Model file for the job. Use its own axes, mm. A direction names the side the tool comes from. Round coordinates to 2 decimals unless told otherwise and drop trailing zeros. Loops run counter-clockwise (first coordinate to the right, second up) from the corner with the lowest first, then second, coordinate; pieces in that order, holes last. Notation, with made-up numbers: M 86.5,-15.5 L 106.5,-15.5 A10 cw 106.5,-8.5 Z; hole C 21,70 d3. An arc over 180 degrees is marked long. Use a Markdown table: item, result. Add a question column.
Q1. Pin check, flat tips, straight feed: pin 1 (2 mm diameter, centred on x = 50, z = 8.5, fed in from -Y); pin 2 (1.4 mm diameter, centred on x = 2, y = 6.5, fed in from +Z); pin 3 (1.6 mm diameter, centred on x = 0.5, z = 12.5, fed in from -Y). Stop position of each tip, or through.
Q2. Cut at A-A (y = 5). Give the cut face in (x, z) (1 decimal).
Q3. Cut at B-B (x = 18). Give the cut face in (y, z), plus the area to 3 significant figures.
Q4. Probe line 1 (X direction, y = 1, z = -0.75); line 2 (Y direction, x = 54, z = -8); line 3 (Y direction, x = 9.5, z = -11). List the from-to ranges inside material, lowest first. Write a range as from..to.
Q5. Tool access for faces 1 (the face through (2, 8, 12)), 2 (the face through (1, 7.3, -12)), 3 (the face through (1, 7.3, 12)): list every direction of +Z, -Z, +X, -X, +Y, -Y with a clear straight run to the whole face (end or side of a thin tool).
Q6. Mould opens along X. For faces 4 (the face through (46.633, 8.243, -0.182)), 5 (the face through (17.99, 12.75, 0.18)), 6 (the face through (60.87, 5.61, 5.48)) say: +X half, -X half, draft (parallel to the pull), parting line (faces both ways), or undercut.
Autodesk Inventor part; units mm, degrees
ref_plane "AK_XY" through (0, -0.05, 0) normal (-1, 0, 0) x (0, 0, -1)
ref_plane "AK_YZ" through (0, -0.05, 0) normal (0, 0, -1) x (0, -1, 0)
ref_plane "AK_ZX" through (0, -0.05, 0) normal (0, -1, 0) x (-1, 0, 0)
sketch "Sketch_26" plane through (0, 0, 0) normal (0, 0, 1) x (1, 0, 0)
  line L0 (0, 15) -> (0, 0)
  line L1 (0, 0) -> (62.6, 0)
  line L2 (62.6, 0) -> (62.6, 15)
  line L3 (62.6, 15) -> (0, 15)
extrude "Extrusion1" add sketch "Sketch_26" along normal mid plane 26
sketch "Sketch_1" plane through (0, 0, 0) normal (1, 0, 0) x (0, 0, -1)
  arc A0 (13, 11.25) -> (-13, 11.25) centre (0, -44.3333) ccw
  line L0 (13, 11.25) -> (13, 20.75)
  line L1 (13, 20.75) -> (-13, 20.75)
  line L2 (-13, 20.75) -> (-13, 11.25)
extrude "Extrusion2" cut sketch "Sketch_1" along normal blind 36.5
sketch "Sketch_12" plane through (0, 13.8, 0) normal (0, 1, 0) x (1, 0, 0)
  line L0 (-1, 16) -> (-1, -14)
  line L1 (-1, -14) -> (64, -14)
  line L2 (64, -14) -> (64, 16)
  line L3 (64, 16) -> (-1, 16)
  line L4 (0, 13) -> (0, -13)
  line L5 (0, -13) -> (36.5, -13)
  arc A0 (36.5, -13) -> (57.121, -8.5497) centre (36.5, 37) ccw
  arc A1 (57.121, -8.5497) -> (57.121, 8.5497) centre (53.2505, 0) ccw
  arc A2 (57.121, 8.5497) -> (36.5, 13) centre (36.5, -37) ccw
  line L6 (36.5, 13) -> (0, 13)
extrude "Extrusion3" cut sketch "Sketch_12" against normal blind 15
sketch "Sketch_3" plane through (36.5, 0, 0) normal (1, 0, 0) x (0, 0, -1)
  line L0 (13, -39.25) -> (-13, -39.25)
  arc A0 (13, 11.25) -> (-13, 11.25) centre (0, -44.3333) ccw
  line L1 (13, 11.25) -> (13, 25.75)
  line L2 (13, 25.75) -> (-13, 25.75)
  line L3 (-13, 25.75) -> (-13, 11.25)
revolve "Revolution1" cut sketch "Sketch_3" angle 35 about axis through (36.5, -39.25, -13) along (0, 0, -1)
sketch "Sketch_2" plane through (0, 0, 0) normal (0, 0, 1) x (1, 0, 0)
  line L0 (0, 7.3) -> (0, -51.7)
  line L1 (0, -51.7) -> (65, -51.7)
  line L2 (65, -51.7) -> (65, 3.3)
  arc A0 (65, 3.3) -> (36.5, 9.3) centre (32.036, -82.5916) ccw
  line L3 (36.5, 9.3) -> (2, 9.3)
  line L4 (2, 9.3) -> (2, 7.3)
  line L5 (2, 7.3) -> (0, 7.3)
extrude "Extrusion4" cut sketch "Sketch_2" along normal mid plane 26
sketch "Sketch_24" plane through (0, 0, 0) normal (0, 0, 1) x (1, 0, 0)
  line L0 (0, 10.75) -> (0, 0)
  line L1 (0, 0) -> (1, 0)
  line L2 (1, 0) -> (1, 3)
  line L3 (1, 3) -> (5.4745, 10.75)
  line L4 (5.4745, 10.75) -> (0, 10.75)
extrude "Extrusion5" add sketch "Sketch_24" along normal mid plane 22
ref_plane "AK_XY" through (0, -0.05, 0) normal (-1, 0, 0) x (0, 0, -1)
ref_plane "AK_YZ" through (0, -0.05, 0) normal (0, 0, -1) x (0, -1, 0)
ref_plane "AK_ZX" through (0, -0.05, 0) normal (0, -1, 0) x (-1, 0, 0)
properties part number "EGC-80-TB-KF_(AK)"
Checked values:
| question | item | result |
|---|---|---|
| 1 | pin 1 | stops at y = 7.43 |
| 1 | pin 2 | stops at z = 11 |
| 1 | pin 3 | stops at y = 7.3 |
| 2 | outline | M 0,-11 L 2.2,-11 L 2.2,11 L 0,11 Z; M 60.2,-6.3 A9.4 ccw 62.6,-0.8 L 62.6,0.8 A9.4 ccw 60.2,6.3 Z |
| 3 | outline | M 9.3,-13 L 11.25,-13 A57.08 ccw 11.25,13 L 9.3,13 Z |
| 3 | area | 76.8 mm^2 |
| 4 | line 1 | x = 0..1 |
| 4 | line 2 | y = 6.75..9.12 |
| 4 | line 3 | y = 9.3..11.68 |
| 5 | face 1 | +Z, -Y |
| 5 | face 2 | -Z, +X, -X, -Y |
| 5 | face 3 | +Z, +X, -X, -Y |
| 6 | face 4 | undercut |
| 6 | face 5 | draft |
| 6 | face 6 | +X half |
